Study the drawing (mm; zero at the part's minimum x, y, z) and answer. A direction names the side the tool comes from. Coordinates: 2 decimals unless noted, no trailing zeros. Loops run counter-clockwise (first coordinate to the right, second up) from the corner with the lowest first, then second, coordinate; pieces in that order, holes last. Notation, with made-up numbers: (43, 66.5) -> (68, 66.5) arc R23 cw to (68, 89.5) -> close; hole circle Ø8 at (35.25, -13). An arc over 180 degrees is marked (long way). Answer in a Markdown table with one row per item.
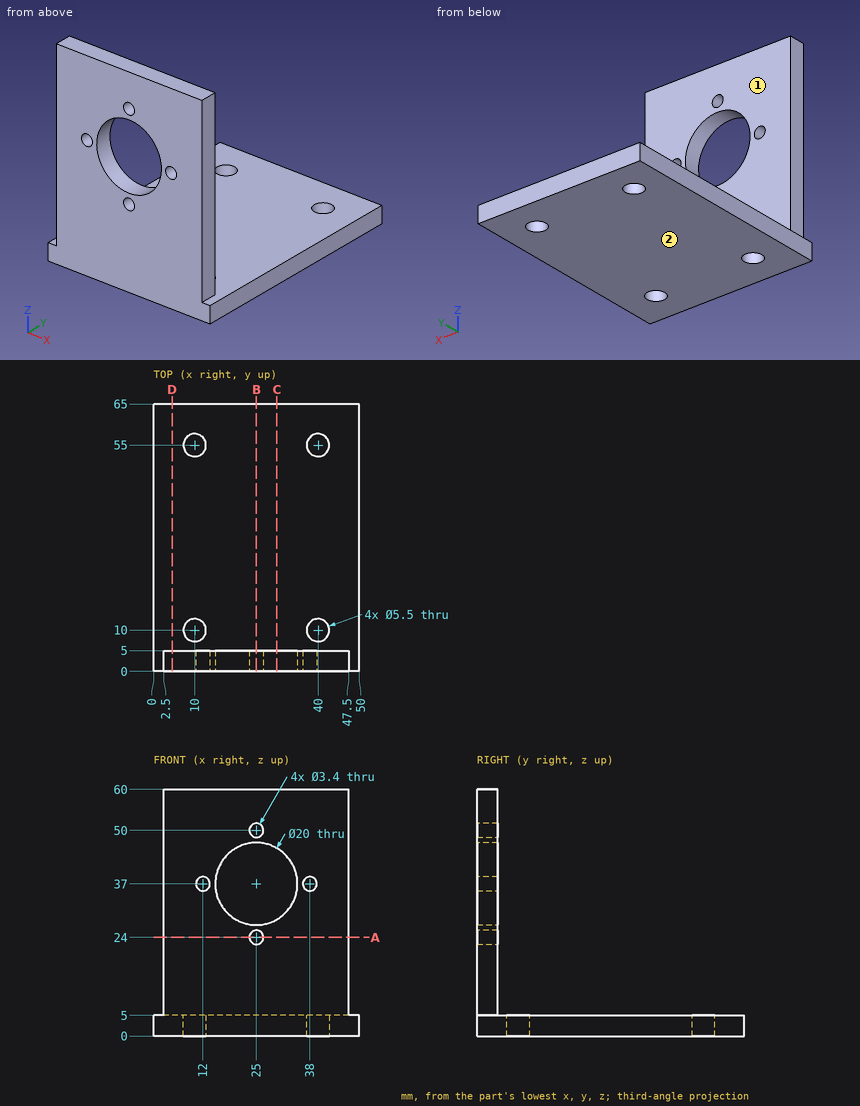
1. Find the intervals of material crossed by probe 1 along X at (y, z) = (1.4, 37); probe 2 along Y at (x, z) = (40, 1); probe 3 along X at (y, z) = (3, 50), in increasing order.
A:
| item | result |
|---|---|
| probe 1 | x = 2.5 to 10.3, 13.7 to 15, 35 to 36.3, 39.7 to 47.5 |
| probe 2 | y = 0 to 7.25, 12.75 to 52.25, 57.75 to 65 |
| probe 3 | x = 2.5 to 23.3, 26.7 to 47.5 |
2. A cutting plane is placed at D-D on x = 4.5. Give the vertices of the cut face in (y, z), and give its area (3 significant figures).
A:
| item | result |
|---|---|
| outline | (0, 0) -> (65, 0) -> (65, 5) -> (5, 5) -> (5, 60) -> (0, 60) -> close |
| area | 600 mm2 |
3. A tool of negligible diameter and unlimited length cuts with its end or side. For the marked faces 1 and 2, from which of +Z, -Z, +X, -X, +Y, -Y can it reach the whole face along a straight path? Write none if from no direction.
A:
| item | result |
|---|---|
| face 1 | +Z, +X, -X, +Y |
| face 2 | -Z, +X, -X, +Y, -Y |
4. A cutting plane is placed at B-B on x = 25. Give the vertices of the cut face in (y, z).
A:
| item | result |
|---|---|
| outline | (0, 0) -> (65, 0) -> (65, 5) -> (5, 5) -> (5, 22.3) -> (0, 22.3) -> close; (0, 25.7) -> (5, 25.7) -> (5, 27) -> (0, 27) -> close; (0, 47) -> (5, 47) -> (5, 48.3) -> (0, 48.3) -> close; (0, 51.7) -> (5, 51.7) -> (5, 60) -> (0, 60) -> close |
5. Given pin 1 Ø6 at (x, y) = (35.5, 12) entering from +Z; pin 2 Ø5.5 at (y, z) = (2, 28) entering from -X; pin 3 Ø16 at (x, z) = (25, 37) entering from -Y; pin 4 Ø4 at (y, z) = (1.5, 29.5) entering from +X, each flat-ended and moving along its own axis, determine where each tip first touches the part or whether it passes through.
A:
| item | result |
|---|---|
| pin 1 | stops at z = 5 |
| pin 2 | stops at x = 2.5 |
| pin 3 | passes through |
| pin 4 | stops at x = 47.5 |
6. A cutting plane is placed at A-A on z = 24. Give the vertices of the cut face in (x, y).
A:
| item | result |
|---|---|
| outline | (2.5, 0) -> (23.3, 0) -> (23.3, 5) -> (2.5, 5) -> close; (26.7, 0) -> (47.5, 0) -> (47.5, 5) -> (26.7, 5) -> close |
7. A cutting plane is placed at C-C on x = 30. Give the vertices of the cut face in (y, z), and give its area (3 significant figures).
A:
| item | result |
|---|---|
| outline | (0, 0) -> (65, 0) -> (65, 5) -> (5, 5) -> (5, 28.34) -> (0, 28.34) -> close; (0, 45.66) -> (5, 45.66) -> (5, 60) -> (0, 60) -> close |
| area | 513 mm2 |
